Geometry check sheet. Reference: the model listing, model coordinates, mm. A direction names the side the tool comes from. Coordinates: 2 decimals unless noted, no trailing zeros. Write each loop counter-clockwise with the first axis right and the second up, starting at its lowest first coordinate (ties: lowest second). Pieces come first, ordered by that corner, then holes.
from build123d import *

# Parameters (mm, degrees)
SKETCH1_R           = 5
SKETCH2_R           = 4.6
SKETCH3_W           = 5.3
SKETCH3_H           = 5.4
BOSS_EXTRUDE1_DEPTH = 8.3
SKETCH4_R           = 1
CUT_EXTRUDE1_DEPTH  = 31.501352471


with BuildPart() as part:
    # Sketch1 → Loft1 section 0
    with BuildSketch(Plane(origin=(0, 0, 0), x_dir=(1, 0, 0), z_dir=(0, 1, 0))):
        Circle(SKETCH1_R)
    # Sketch2 → Loft1 section 1
    with BuildSketch(Plane(origin=(0, 20.8, 0), x_dir=(1, 0, 0), z_dir=(0, 1, 0))):
        Circle(SKETCH2_R)
    loft()

    # Sketch3 → Boss-Extrude1 (add)
    with BuildSketch(Plane(origin=(0, 20.8, 0), x_dir=(1, 0, 0), z_dir=(0, 1, 0))):
        Rectangle(SKETCH3_W, SKETCH3_H)
    extrude(amount=BOSS_EXTRUDE1_DEPTH)

    # Sketch4 → Cut-Extrude1 (cut, through all)
    with BuildSketch(Plane.ZY.offset(2.65)):
        with Locations((0, 25.95)):
            Circle(SKETCH4_R)
    extrude(amount=-CUT_EXTRUDE1_DEPTH, mode=Mode.SUBTRACT)


solid = part.part
1. Sectioned sample at A-A, the plane y = 26.25. Record the boundary of the cut face in (x, z), and give its area (3 significant figures).
Computed values:
outline: (-2.65, -2.7) - (2.65, -2.7) - (2.65, -0.95) - (-2.65, -0.95) - close; (-2.65, 0.95) - (2.65, 0.95) - (2.65, 2.7) - (-2.65, 2.7) - close
area: 18.5 mm2
2. Draft check along Z on faces 5 (the cylindrical face through (-0.04, 25.06, 0.46)), 6 (the flat face through (0, 25, 2.7)), 7 (the flat face through (0, 29.1, 0)). Enter one of: released by +Z, released by -Z, zero draft, split by the parting line, or undercut.
Computed values:
face 5: undercut
face 6: released by +Z
face 7: zero draft
3. Gauge pin test, flat ends, axial feed: pin 1 Ø6 at (x, y) = (4, 8) entering from +Z; pin 2 Ø6 at (x, y) = (1, 7.5) entering from +Z; pin 3 Ø2.5 at (y, z) = (23.5, 0.5) entering from +X. Record the tip position at first contact, or that the pin passes through.
Computed values:
pin 1: stops at z = 4.74
pin 2: stops at z = 4.91
pin 3: stops at x = 2.65
4. Thickness scan on line 1 along Y through (x, z) = (1.1, 0); line 2 along X through (y, z) = (19.75, -3.75); line 3 along Y through (x, z) = (-2.5, 3). Record the ranges inside material, lowest first.
Computed values:
line 1: y = 0 to 24.95, 26.95 to 29.1
line 2: x = -2.7 to 2.7
line 3: y = 0 to 20.8
5. Access from +Z, -Z, +X, -X, +Y, -Y to the whole of each face (thin tool, end or side, straight path). Record for faces 1 (the flat face through (-2.65, 25, 1)), 2 (the conical face through (-1.04, 10.546, 4.683)), 3 (the flat face through (2.65, 25, 1)), 4 (the flat face through (0, 25, -2.7)).
Computed values:
face 1: +Z, -Z, -X, +Y
face 2: +Y
face 3: +Z, -Z, +X, +Y
face 4: -Z, +X, -X, +Y
6. Sectioned sample at B-B, the plane y = 21.25. Record the boundary of the cut face in (x, z), and give its area (3 significant figures).
Computed values:
outline: (-2.65, -2.7) - (2.65, -2.7) - (2.65, 2.7) - (-2.65, 2.7) - close
area: 28.6 mm2
